Source: CAD feature listing. Evaluate the final solid. Frame: model axes, mm. Face numbers are marked on the shaded views. Give positions to 0.01 mm unless a question says otherwise; leave off trailing zeros. Loops run counter-clockwise (first coordinate to the right, second up) from the corner with the lowest first, then second, coordinate; pieces in that order, holes last. Notation, with made-up numbers: (81.5, 20.25) -> (129.5, 20.25) arc R15 ccw to (129.5, 39.25) -> close; hole circle Ø11 at (29, 12). An arc over 180 degrees is marked (long way). Put each result on its own line as item: value.
```python
from build123d import *

# Parameters (mm, degrees)
REVOLVE1_START         = 5.08
REVOLVE1_OUTLINE_R     = 18.161
REVOLVE1_OUTLINE_R_2   = 16.891
REVOLVE1_DEPTH         = 253.238
REVOLVE1_2_OUTLINE_R   = 20.701
REVOLVE1_2_OUTLINE_R_2 = 18.161
REVOLVE1_2_DEPTH       = 7.62
CUT_EXTRUDE1_DEPTH     = 5.08
CIRPATTERN1_COUNT      = 3


# Read off the part's stored shape, not the designer's step: Revolve1
with BuildPart() as part:
    # Revolve1 outline → Revolve1 (new body)
    with BuildSketch(Plane.YZ.offset(REVOLVE1_START)):
        Circle(REVOLVE1_OUTLINE_R)
        Circle(REVOLVE1_OUTLINE_R_2, mode=Mode.SUBTRACT)
    extrude(amount=REVOLVE1_DEPTH)

    # Revolve1 2 outline → Revolve1 2 (add)
    with BuildSketch(Plane.YZ):
        Circle(REVOLVE1_2_OUTLINE_R)
        Circle(REVOLVE1_2_OUTLINE_R_2, mode=Mode.SUBTRACT)
    extrude(amount=REVOLVE1_2_DEPTH)

    # Sketch2 → Cut-Extrude1 (cut)
    with BuildSketch(Plane(origin=(0, 18.161, 0), x_dir=(1, 0, 0), z_dir=(0, 1, 0))):
        with BuildLine():
            Line((20.6375, 3.175), (20.6375, -3.175))
            ThreePointArc((20.6375, -3.175), (19.05, -4.7625), (17.4625, -3.175))
            Line((17.4625, -3.175), (17.4625, 3.175))
            ThreePointArc((17.4625, 3.175), (19.05, 4.7625), (20.6375, 3.175))
        make_face()
    cut_extrude1 = extrude(amount=-CUT_EXTRUDE1_DEPTH, mode=Mode.SUBTRACT)

    # CirPattern1: Cut-Extrude1 ×3 about axis
    cirpattern1_axis = Axis((0, 0, 0), (-1, 0, 0))
    for i in range(1, CIRPATTERN1_COUNT):
        add(cut_extrude1.rotate(cirpattern1_axis, i * 360 / CIRPATTERN1_COUNT), mode=Mode.SUBTRACT)


solid = part.part
```
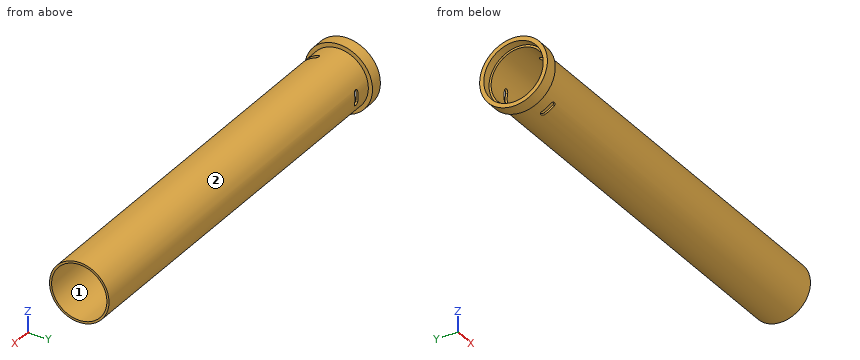
(1) Section B-B on y = 0. Return loops of the section in (x, z), then the cut area to 3 significant figures.
Calculated:
outline: (0, -20.7) -> (7.62, -20.7) -> (7.62, -18.16) -> (258.32, -18.16) -> (258.32, -16.89) -> (5.08, -16.89) -> (5.08, -18.16) -> (0, -18.16) -> close; (0, 18.16) -> (5.08, 18.16) -> (5.08, 16.89) -> (258.32, 16.89) -> (258.32, 18.16) -> (7.62, 18.16) -> (7.62, 20.7) -> (0, 20.7) -> close
area: 682 mm²
(2) Draft query along Z for the marked faces 1 and 2. Return one class per face: released by +Z, released by -Z, zero draft, split by the parting line, or undercut.
Calculated:
face 1: undercut
face 2: split by the parting line
(3) First-contact query: P1, Ø11, axis at y = -5, z = -8.5, coming from the -X side; P2, Ø6, axis at x = 38.5, y = -11, coming from the +Z side; P3, Ø6, axis at x = 29.5, y = -14.5, coming from the -Z side; P4, Ø1, axis at x = 120.5, y = -10.5, coming from the +Z side. Flat tips, straight axial feed; report the tip coordinate or a pass-through.
Calculated:
P1: passes through
P2: stops at z = 16.3
P3: stops at z = -14.06
P4: stops at z = 15.16
(4) Line query: probe 1 along Z at (x, y) = (59.5, 0); probe 2 along Z at (x, y) = (57, -4.5); probe 3 along X at (y, z) = (-18.5, 3.5). Output: solid intervals per line, ascending. Write a range as from..to.
Calculated:
probe 1: z = -18.16..-16.89, 16.89..18.16
probe 2: z = -17.59..-16.28, 16.28..17.59
probe 3: x = 0..7.62
(5) Section A-A on z = 0. Return loops of the section in (x, y).
Calculated:
outline: (0, -20.7) -> (7.62, -20.7) -> (7.62, -18.16) -> (258.32, -18.16) -> (258.32, -16.89) -> (5.08, -16.89) -> (5.08, -18.16) -> (0, -18.16) -> close; (0, 18.16) -> (5.08, 18.16) -> (5.08, 16.89) -> (17.46, 16.89) -> (17.46, 18.16) -> (7.62, 18.16) -> (7.62, 20.7) -> (0, 20.7) -> close; (20.64, 16.89) -> (258.32, 16.89) -> (258.32, 18.16) -> (20.64, 18.16) -> close
(6) Section C-C on x = 39.5. Return loops of the section in (y, z).
Calculated:
outline: circle Ø36.32 at (0, 0); hole circle Ø33.78 at (0, 0)
